Source: CAD feature listing. Evaluate the final solid. Frame: model axes, mm. A direction names the side the tool comes from. Coordinates: 2 decimals unless noted, no trailing zeros. Loops run counter-clockwise (first coordinate to the right, second up) from the corner with the lowest first, then second, coordinate; pieces in that order, holes last. Notation, with made-up numbers: (75.25, 18) - (96.25, 18) arc R24 ccw to (96.25, 46) - close; hole circle Ø6 at (-26.5, 70). An arc over 180 degrees is marked (long way). Use one line per item in the form item = value. Start each with the question number.
from build123d import *

# Parameters (mm, degrees)
F0_R         = 20
F1_DEPTH     = 12
F3_D         = 3.1
F3_DEPTH     = 8
F3_TIP       = 0.9313339595
F5_DEPTH     = 12.001
F6_W         = 5
F6_H         = 10.46546828
F7_DEPTH     = 12
F8_W         = 2
F8_H         = 10.46546828
F9_DEPTH     = 11
F10_W        = 1
F10_H        = 10.46546828
F11_DEPTH    = 5
F12_T1_DEPTH = 10.46546828
F12_T3_DEPTH = 10.46546828


# Not quite as in the source:
# - a fillet or chamfer that OpenCascade refuses, or shapes differently, is made with other operations: its cross-section is extruded or revolved along the edge and cut away or added


with BuildPart() as f1:
    # F0 (on Top) → F1 (new body)
    with BuildSketch(Plane.XY):
        Circle(F0_R)
    extrude(amount=F1_DEPTH)

    # F3
    with Locations(Plane(origin=(0, 0, 0), x_dir=(1, 0, 0), z_dir=(0, 0, -1))):
        with Locations((-10.9601551084, 10.9601551084), (-10.9601551084, -10.9601551084), (10.9601551084, -10.9601551084), (10.9601551084, 10.9601551084)):
            Hole(F3_D / 2, depth=F3_DEPTH)
            with Locations((0, 0, -(F3_DEPTH + F3_TIP / 2))):  # 118° drill point
                Cone(0, F3_D / 2, F3_TIP, mode=Mode.SUBTRACT)

    # F4 (on face) → F5 (intersect, through all)
    with BuildSketch(Plane.XY.offset(12)):
        with BuildLine():
            Line((13, -7), (13, 7))
            Line((13, 7), (18.7349939952, 7))
            ThreePointArc((18.7349939952, 7), (0, 20), (-18.7349939952, 7))
            Line((-18.7349939952, 7), (-13, 7))
            Line((-13, 7), (-13, -7))
            Line((-13, -7), (-18.7349939952, -7))
            ThreePointArc((-18.7349939952, -7), (0, -20), (18.7349939952, -7))
            Line((18.7349939952, -7), (13, -7))
        make_face()
    extrude(amount=-F5_DEPTH, mode=Mode.INTERSECT)

    # F6 (on Top) → F7 (join)
    with BuildSketch(Plane.XY):
        with Locations((15.5, 0)):
            Rectangle(F6_W, F6_H)
    extrude(amount=F7_DEPTH)

    # F8 (on face) → F9 (cut)
    with BuildSketch(Plane.XY.offset(12)):
        with Locations((16, 0)):
            Rectangle(F8_W, F8_H)
    extrude(amount=-F9_DEPTH, mode=Mode.SUBTRACT)

    # F10 (on Top) → F11 (cut)
    with BuildSketch(Plane.XY):
        with Locations((13.5, 0)):
            Rectangle(F10_W, F10_H)
    extrude(amount=F11_DEPTH, mode=Mode.SUBTRACT)

    # F12: fillet of radius 1 on 6 edges, made by hand

    # F12_s2 → F12_t1 (join)
    with BuildSketch(Plane.XZ.offset(-5.23273414)):
        with BuildLine():
            ThreePointArc((15, 2), (15.2928932188, 1.2928932188), (16, 1))
            Line((16, 1), (15, 1))
            Line((15, 1), (15, 2))
        make_face()
        with BuildLine():
            ThreePointArc((16, 1), (16.7071067812, 1.2928932188), (17, 2))
            Line((17, 2), (17, 1))
            Line((17, 1), (16, 1))
        make_face()
        with BuildLine():
            ThreePointArc((14, 4), (13.7071067812, 4.7071067812), (13, 5))
            Line((13, 5), (14, 5))
            Line((14, 5), (14, 4))
        make_face()
        with BuildLine():
            ThreePointArc((13, 4), (13.2928932188, 4.7071067812), (14, 5))
            Line((14, 5), (13, 5))
            Line((13, 5), (13, 4))
        make_face()
    extrude(amount=F12_T1_DEPTH)

    # F12_s4 → F12_t3 (cut)
    with BuildSketch(Plane.XZ.offset(-5.23273414)):
        with BuildLine():
            ThreePointArc((18, 1), (17.7071067812, 0.2928932188), (17, 0))
            Line((17, 0), (18, 0))
            Line((18, 0), (18, 1))
        make_face()
        with BuildLine():
            ThreePointArc((14, 1), (14.2928932188, 0.2928932188), (15, 0))
            Line((15, 0), (14, 0))
            Line((14, 0), (14, 1))
        make_face()
    extrude(amount=F12_T3_DEPTH, mode=Mode.SUBTRACT)


solid = f1.part
(1) Mould query, pull axis X, two halves, no side actions, for faces 1 (the face through (-12.439, -11.426, 4.056)), 2 (the face through (0, -20, 6)), 3 (the face through (-16, 7, 6)), 4 (the face through (-13, 0, 6)). Classes: +X half, -X half, draft (parallel to the pull), parting line (faces both ways), or undercut.
(2) Cut plane D-D, the plane z = 11. Output: boundary loops of the cut face in (x, y) (3 decimals).
(3) Material intervals for line 1 (X direction, y = -3.5, z = 8.75); line 2 (Y direction, x = 11.5, z = 3.75); line 3 (X direction, y = 11, z = 7.5), sorted ascending.
(4) Contact query for flat-ended pins moving along their axis: pin 1 (1.5 mm diameter, centred on y = 2.5, z = 4.5, fed in from -X); pin 2 (6 mm diameter, centred on y = -2, z = 8, fed in from +X); pin 3 (1 mm diameter, centred on x = 6.5, z = 1.5, fed in from -Y). Output: stop coordinate, or through.
(5) Cut plane C-C, the plane z = 3. Output: boundary loops of the cut face in (x, y) (3 decimals).
(6) Cut plane A-A, the plane z = 7.5. Output: boundary loops of the cut face in (x, y) (3 decimals).
(7) Access query for faces 5 (the face through (17.715, 0.073, 0.301)), 6 (the face through (13, 0, 3)), 7 (the face through (16, 7, 6)), 8 (the face through (-16, -7, 6)). Directions: +Z, -Z, +X, -X, +Y, -Y. A direction counts if a zero-diameter tool reaches every point of the face in a straight line with its end or side. Return the directions, or none.
(8) Cut plane B-B, the plane y = -4. Output: boundary loops of the cut face in (x, z).
Recorded:
q1.face_1 = undercut
q1.face_2 = parting line
q1.face_3 = draft
q1.face_4 = -X half
q2.outline = (-18.735, -7) arc R20 ccw to (18.735, -7) - (13, -7) - (13, -5.233) - (15, -5.233) - (15, 5.233) - (13, 5.233) - (13, 7) - (18.735, 7) arc R20 ccw to (-18.735, 7) - (-13, 7) - (-13, -7) - close; (17, -5.233) - (18, -5.233) - (18, 5.233) - (17, 5.233) - close
q3.line_1 = -13 to 15, 17 to 18
q3.line_2 = -16.36 to -12.41, -9.51 to 9.51, 12.41 to 16.36
q3.line_3 = -16.7 to -12.51, -9.41 to 9.41, 12.51 to 16.7
q4.pin_1 = -13
q4.pin_2 = 18
q4.pin_3 = -19.08
q5.outline = (-18.735, -7) arc R20 ccw to (18.735, -7) - (13, -7) - (13, 7) - (18.735, 7) arc R20 ccw to (-18.735, 7) - (-13, 7) - (-13, -7) - close; (14, -5.233) - (15, -5.233) - (15, 5.233) - (14, 5.233) - close; (17, -5.233) - (18, -5.233) - (18, 5.233) - (17, 5.233) - close; hole circle Ø3.1 at (-10.96, -10.96); hole circle Ø3.1 at (-10.96, 10.96); hole circle Ø3.1 at (10.96, -10.96); hole circle Ø3.1 at (10.96, 10.96)
q6.outline = (-18.735, -7) arc R20 ccw to (18.735, -7) - (13, -7) - (13, -5.233) - (15, -5.233) - (15, 5.233) - (13, 5.233) - (13, 7) - (18.735, 7) arc R20 ccw to (-18.735, 7) - (-13, 7) - (-13, -7) - close; (17, -5.233) - (18, -5.233) - (18, 5.233) - (17, 5.233) - close; hole circle Ø3.1 at (-10.96, -10.96); hole circle Ø3.1 at (-10.96, 10.96); hole circle Ø3.1 at (10.96, -10.96); hole circle Ø3.1 at (10.96, 10.96)
q7.face_5 = -Z, +X
q7.face_6 = -Z
q7.face_7 = +Z, -Z, +X
q7.face_8 = +Z, -Z, -X
q8.outline = (-13, 0) - (13, 0) - (13, 4) arc R1 cw to (13.5, 4.87) arc R1 cw to (14, 4) - (14, 1) arc R1 ccw to (15, 0) - (17, 0) arc R1 ccw to (18, 1) - (18, 12) - (17, 12) - (17, 2) arc R1 cw to (15, 2) - (15, 12) - (-13, 12) - close
